The model under review builds one solid part; all positions refer to its coordinate system, in mm. Round coordinates to 2 decimals unless told otherwise and drop trailing zeros. Loops run counter-clockwise (first coordinate to the right, second up) from the corner with the lowest first, then second, coordinate; pieces in that order, holes last. Notation, with made-up numbers: M 77.25,-27.5 L 136.25,-27.5 A35 cw 136.25,4.5 Z; hole C -21,-29 d11. An arc over 180 degrees is marked long. Return JSON: item names as keys, results as strings. Group by question number.
Q1. To check wall thickness, follow line 1 along Z through (x, y) = (0, -0.1); line 2 along X through (y, z) = (-0.2, -28.5); line 3 along X through (y, z) = (-0.25, -30.5). State the ranges of each line that lie inside material, in increasing order.
Q2. Draft analysis for pull direction Z (two halves, no side actions). For faces 1 (the face through (34.834, -0.246, -35.063)), 2 (the face through (0.36, -0.25, 42.47)), 3 (the face through (-0.36, -0.25, -42.45)), 4 (the face through (-38, -0.5, 0)), state which applies: pulls with the +Z half, pulls with the -Z half, needs draft (parallel to the pull), parting line crosses it, or undercut.
Q3. Consider section D-D (y = -0.1). State the section outline as (x, z) points, and give its area (3 significant figures).
Q4. Consider section B-B (z = 0). State the section outline as (x, y) points.
Q5. Consider section C-C (x = -30). State the section outline as (y, z) points, and give its area (3 significant figures).
Q6. Consider section A-A (x = 0). State the section outline as (y, z) points.
from build123d import *

# Parameters (mm, degrees)
F0_R     = 3
F0_R_2   = 37.5
F1_DEPTH = 0.5


with BuildPart() as f1:
    # F0 (on Front) → F1 (new body)
    with BuildSketch(Plane.XZ):
        with BuildLine():
            ThreePointArc((24.65233, 34.529271), (-0.003968, 42.471267), (-24.658782, 34.524663))
            ThreePointArc((-24.658782, 34.524663), (-34.949737, 34.94989), (-34.524555, 24.658933))
            ThreePointArc((-34.524555, 24.658933), (-42.417707, 0), (-34.524555, -24.658933))
            ThreePointArc((-34.524555, -24.658933), (-34.911112, -34.91779), (-24.65233, -34.529271))
            ThreePointArc((-24.65233, -34.529271), (0.003966, -42.451585), (24.658782, -34.524663))
            ThreePointArc((24.658782, -34.524663), (34.949737, -34.94989), (34.524555, -24.658933))
            ThreePointArc((34.524555, -24.658933), (42.374192, 0), (34.524555, 24.658933))
            ThreePointArc((34.524555, 24.658933), (34.911112, 34.91779), (24.65233, 34.529271))
        make_face()
        with Locations((-29.961838, -29.967569)):
            Circle(F0_R, mode=Mode.SUBTRACT)
        with Locations((30, -30.000132)):
            Circle(F0_R, mode=Mode.SUBTRACT)
        Circle(F0_R_2, mode=Mode.SUBTRACT)
        with Locations((-30, 30.000132)):
            Circle(F0_R, mode=Mode.SUBTRACT)
        with Locations((29.961838, 29.967569)):
            Circle(F0_R, mode=Mode.SUBTRACT)
    extrude(amount=F1_DEPTH)


solid = f1.part
Values:
{
 "1": {"line 1": "z = -42.45 to -37.5, 37.5 to 42.47", "line 2": "x = -36.81 to -32.58, -27.35 to -24.37, 24.37 to 27.4, 32.6 to 36.84", "line 3": "x = -36.94 to -32.91, -27.01 to -21.82, 21.82 to 27.04, 32.96 to 36.98"},
 "2": {"face 1": "undercut", "face 2": "pulls with the +Z half", "face 3": "pulls with the -Z half", "face 4": "needs draft"},
 "3": {"outline": "M -34.52,-24.66 A7 ccw long -24.65,-34.53 A42.32 ccw 24.66,-34.52 A7 ccw long 34.52,-24.66 A42.66 ccw 34.52,24.66 A7 ccw long 24.65,34.53 A42.23 ccw -24.66,34.52 A7 ccw long -34.52,24.66 A42.46 ccw Z; hole C 0,0 d75; hole C -30,30 d6; hole C -29.96,-29.97 d6; hole C 29.96,29.97 d6; hole C 30,-30 d6", "area": "1,440 mm2"},
 "4": {"outline": "M -42.42,-0.5 L -37.5,-0.5 L -37.5,0 L -42.42,0 Z; M 37.5,-0.5 L 42.37,-0.5 L 42.37,0 L 37.5,0 Z"},
 "5": {"outline": "M -0.5,-36.97 L 0,-36.97 L 0,-32.97 L -0.5,-32.97 Z; M -0.5,-26.97 L 0,-26.97 L 0,-22.5 L -0.5,-22.5 Z; M -0.5,22.5 L 0,22.5 L 0,27 L -0.5,27 Z; M -0.5,33 L 0,33 L 0,37 L -0.5,37 Z", "area": "8.48 mm2"},
 "6": {"outline": "M -0.5,-42.45 L 0,-42.45 L 0,-37.5 L -0.5,-37.5 Z; M -0.5,37.5 L 0,37.5 L 0,42.47 L -0.5,42.47 Z"}
}
